Autodesk Inventor part; units mm, degrees
ref_plane "YZ Plane" through (0, 0, 0) normal (1, 0, 0) x (0, 1, 0)
ref_plane "XZ Plane" through (0, 0, 0) normal (0, 1, 0) x (-1, 0, 0)
ref_plane "XY Plane" through (0, 0, 0) normal (0, 0, 1) x (1, 0, 0)
sketch "Sketch1" plane through (0, 0, 0) normal (0, 0, 1) x (1, 0, 0)
  circle A0 centre (0, 0) radius 25
  dimension "d0" = 50
extrude "Extrusion1" add sketch "Sketch1" along normal blind 36
sketch "Sketch2" plane through (0, 0, 36) normal (0, 0, 1) x (1, 0, 0)
  circle A0 centre (0, 0) radius 24
  dimension "d3" = 48
extrude "Extrusion2" add sketch "Sketch2" along normal blind 5
sketch "Sketch3" plane through (0, 0, 0) normal (0, 0, -1) x (-1, 0, 0)
  circle A0 centre (0, 0) radius 24
  dimension "d6" = 48
extrude "Extrusion3" add sketch "Sketch3" along normal blind 26
sketch "Sketch4" plane through (0, 0, 41) normal (0, 0, 1) x (1, 0, 0)
  circle A0 centre (0, 0) radius 9
  dimension "d9" = 18
extrude "Extrusion4" add sketch "Sketch4" along normal blind 5
sketch "Sketch5" plane through (0, 0, 46) normal (0, 0, 1) x (1, 0, 0)
  circle A0 centre (0, 0) radius 2.5
  dimension "d12" = 5
extrude "Extrusion5" add sketch "Sketch5" along normal blind 14
sketch "Sketch6" plane through (0, 0, 41) normal (0, 0, 1) x (1, 0, 0)
  circle A0 centre (0, 0) radius 2.5
  circle A1 centre (0, 0) radius 16
  circle A2 centre (16, 0) radius 2.5
  circle A3 centre (0, 16) radius 2.5
  circle A4 centre (-16, 0) radius 2.5
  circle A5 centre (0, -16) radius 2.5
  dimension "d15" = 32
  dimension "d16" = 5
  dimension "d19" = 360
extrude "Extrusion6" cut sketch "Sketch6" against normal blind 10 contours A1 A2 | A1 A2 | A3 A1 | A1 A3 | A5 A1 | A1 A5 | A4 A1 | A1 A4
properties part number "MOTOR 895"
The model under review builds one solid part; all positions refer to its coordinate system, in mm. A direction names the side the tool comes from. Give positions to 0.01 mm unless a question says otherwise; leave off trailing zeros. Write each loop counter-clockwise with the first axis right and the second up, starting at its lowest first coordinate (ties: lowest second). Pieces come first, ordered by that corner, then holes. Notation, with made-up numbers: M 60.25,6.25 L 81.25,6.25 A33 ccw 81.25,45.25 Z; hole C 28.25,-9 d3. An arc over 180 degrees is marked long. Write each question's results on one line, items separated by ' | '. Start each with the question number.
1. We need section C-C (z = -17.5). Write out the cut boundary in (x, y).
2. We need section A-A (y = 0). Write out the cut boundary in (x, z), and give its area (3 significant figures).
3. We need section D-D (y = 6). Write out the cut boundary in (x, z), and give its area (3 significant figures).
4. Insertion check: pin 1 Ø5.5 at (x, y) = (0.5, 17) entering from +Z; pin 2 Ø10 at (x, z) = (2, -8.5) entering from -Y; pin 3 Ø12 at (x, z) = (0, -2) entering from -Y. Each pin has a flat end and moves straight along its axis. Give the tip position at first contact, or say it passes through.
5. For probe 1 along Y at (x, z) = (0, 33); probe 2 along Y at (x, z) = (0, 38.75); probe 3 along Z at (x, y) = (16, 17), list the stretches that pass through material, from the lowest coordinate up. Write a range as [from, to].
6. Mouldability with a two-part tool opening along X and no side actions: class faces 1 (the flat face through (0, 16, 31)), 2 (the flat face through (-9.4, 22.3, 36)), 3 (the cylindrical face through (-1.172, -8.923, 43.465)) as released by +X, released by -X, zero draft, split by the parting line, or undercut.
7. For faces 4 (the flat face through (0, 0, 60)), 5 (the flat face through (16, 0, 31)), 6 (the cylindrical face through (23.977, -1.055, -12.818)), list the 3-axis set-ups (+Z, -Z, +X, -X, +Y, -Y) from which the entire face can be reached by the end or side of a thin tool; tool diameter is ignored.
Results found:
1) outline: C 0,0 d48
2) outline: M -25,0 L -24,0 L -24,-26 L 24,-26 L 24,0 L 25,0 L 25,36 L 24,36 L 24,41 L 18.5,41 L 18.5,31 L 13.5,31 L 13.5,41 L 9,41 L 9,46 L 2.5,46 L 2.5,60 L -2.5,60 L -2.5,46 L -9,46 L -9,41 L -13.5,41 L -13.5,31 L -18.5,31 L -18.5,41 L -24,41 L -24,36 L -25,36 Z | area: 3,350 mm^2
3) outline: M -24.27,0 L -23.24,0 L -23.24,-26 L 23.24,-26 L 23.24,0 L 24.27,0 L 24.27,36 L 23.24,36 L 23.24,41 L 6.71,41 L 6.71,46 L -6.71,46 L -6.71,41 L -23.24,41 L -23.24,36 L -24.27,36 Z | area: 3,260 mm^2
4) pin 1: stops at z = 41 | pin 2: stops at y = -24 | pin 3: stops at y = -25
5) probe 1: y = [-25, -18.5], [-13.5, 13.5], [18.5, 25] | probe 2: y = [-24, -18.5], [-13.5, 13.5], [18.5, 24] | probe 3: z = [-26, 41]
6) face 1: undercut | face 2: zero draft | face 3: split by the parting line
7) face 4: +Z, +X, -X, +Y, -Y | face 5: +Z | face 6: -Z
